Design review of the part built by this model. Coordinates are the model's own, in mm. A direction names the side the tool comes from. Round coordinates to 2 decimals unless told otherwise and drop trailing zeros. Write each loop counter-clockwise with the first axis right and the second up, starting at its lowest first coordinate (ties: lowest second). Pieces come first, ordered by that corner, then holes. Notation, with made-up numbers: M 52.5,-38 L 93.5,-38 A37 ccw 93.5,0 Z; hole C 0.25,32 d1. An arc over 180 degrees is marked long. Use CSV: the item, a comma, the result in double quotes.
from build123d import *

# Parameters (mm, degrees)
BOSS_EXTRUDE1_DEPTH = 17
BOSS_EXTRUDE2_DEPTH = 3


with BuildPart() as part:
    # Sketch1 → Boss-Extrude1 (new body, symmetric)
    with BuildSketch(Plane(origin=(0, 0, 0), x_dir=(0, 0, -1), z_dir=(1, 0, 0))):
        Polygon((-7.5, -5), (7.5, -5), (7.5, 5), align=None)
    extrude(amount=BOSS_EXTRUDE1_DEPTH, both=True)

    # Sketch2 → Boss-Extrude2 (add)
    with BuildSketch(Plane(origin=(17, 0, 0), x_dir=(0, 0, -1), z_dir=(1, 0, 0))):
        Polygon((-7.5, -5), (-7.5, 2.722617257), (7.5, 12.722617257), (7.5, -5), align=None)
    boss_extrude2 = extrude(amount=BOSS_EXTRUDE2_DEPTH)

    # Mirror1: Boss-Extrude2 across plane
    add(boss_extrude2.mirror(Plane(origin=(0, 0, 0), x_dir=(0, 0, 1), z_dir=(1, 0, 0))))


solid = part.part
1) Machinability: for faces 1 (the face through (17, 4, 0)), 2 (the face through (0, 2, -7.5)), which of the approach directions +Z, -Z, +X, -X, +Y, -Y give a long, thin tool a straight path to every point of the face, cutting with its end or side? Answer none if there is none.
Answers:
face 1,"+Z, +Y"
face 2,"-Z, +X, -X, +Y, -Y"
2) Add section C-C on z = 5.5. Write out the cut boundary in (x, y).
Answers:
outline,"M -20,-5 L 20,-5 L 20,4.06 L 17,4.06 L 17,-3.67 L -17,-3.67 L -17,4.06 L -20,4.06 Z"
3) Add section D-D on x = 16.5. Write out the cut boundary in (y, z).
Answers:
outline,"M -5,-7.5 L 5,-7.5 L -5,7.5 Z"
4) Wall thickness on line 1 along X through (y, z) = (5.5, 0.5); line 2 along Y through (x, z) = (6.5, -1.5); line 3 along Z through (x, y) = (7.5, 3.25) (3 decimals): over which ranges is each line inside the solid? List them lowest first. Write a range as [from, to].
Answers:
line 1,"[-20, -17], [17, 20]"
line 2,"[-5, 1]"
line 3,"[-7.5, -4.875]"
5) Add section B-B on y = 0.5. Write out the cut boundary in (x, z).
Answers:
outline,"M -20,-7.5 L 20,-7.5 L 20,7.5 L 17,7.5 L 17,-0.75 L -17,-0.75 L -17,7.5 L -20,7.5 Z"
6) The part is to be moulded in two halves that separate along X. For faces 3 (the face through (-20, 2, -2)), 4 (the face through (0, 0, 0)), 5 (the face through (-18, -1, 7.5)), say which applies: released by +X, released by -X, zero draft, split by the parting line, or undercut.
Answers:
face 3,"released by -X"
face 4,"undercut"
face 5,"zero draft"
7) Add section A-A on y = 7.25. Write out the cut boundary in (x, z), then the cut area to 3 significant figures.
Answers:
outline,"M -20,-7.5 L -17,-7.5 L -17,0.71 L -20,0.71 Z; M 17,-7.5 L 20,-7.5 L 20,0.71 L 17,0.71 Z"
area,"49.3 mm²"
8) For pin 1 Ø1 at (x, z) = (6.5, -3.5) entering from +Y; pin 2 Ø3 at (x, y) = (12, 5) entering from +Z; pin 3 Ø5 at (x, z) = (2.5, 0.5) entering from +Y, all flat-tipped, find the tip position at first contact; note any pin that passes through.
Answers:
pin 1,"y = 2.67"
pin 2,"z = -5.25"
pin 3,"y = 1.33"
